Geometry check sheet. Reference: the model listing, model coordinates, mm. A direction names the side the tool comes from. Give positions to 0.01 mm unless a question says otherwise; leave off trailing zeros. Loops run counter-clockwise (first coordinate to the right, second up) from the corner with the lowest first, then second, coordinate; pieces in that order, holes last. Notation, with made-up numbers: (82, -38.75) -> (93, -38.75) arc R5 cw to (93, -29.75) -> close; hole circle Ø5 at (-31.75, -32). An arc over 180 degrees is marked (long way). Write each question's results on one line, items separated by ' | '. Start each with the question number.
1) Depth check by flat-ended pin: pin 1 (9 mm diameter, centred on x = 23, z = -14, fed in from -Y); pin 2 (1 mm diameter, centred on x = 18.5, y = -13.5, fed in from -Z); pin 3 (8 mm diameter, centred on x = 5.5, z = -12, fed in from -Y). Enter the tip coordinate at first touch or a pass-through.
2) Draft check along Z on faces 3 (the face through (18.36, -16.41, -9.74)), 4 (the face through (20, 0, -14)), 5 (the face through (18.95, -21.32, -17.1)). Enter one of: pulls with the +Z half, pulls with the -Z half, needs draft (parallel to the pull), parting line crosses it, or undercut.
3) Sectioned sample at B-B on y = -8.25. Record the cut outline in (x, z).
4) Sectioned sample at C-C on z = -14. Record the cut outline in (x, y).
5) Scan lines: line 1 (Y direction, x = 3, z = -13.5); line 2 (Y direction, x = 11.5, z = -16.5); line 3 (Z direction, x = 23, y = -20). Record each from-to range of solid material in increasing order. Write a range as from..to.
6) Sectioned sample at D-D on x = 23. Record the cut outline in (y, z).
7) Set-up check for faces 1 (the face through (0, -5, -14)), 2 (the face through (7, -7.8, -14)): record each of +Z, -Z, +X, -X, +Y, -Y from which the full face is reachable in a straight line by a thin tool's end or side.
8) Sectioned sample at A-A on x = 7. Record the cut outline in (y, z).
```python
from build123d import *

# Parameters (mm, degrees)
F0_W     = 40.5
F0_H     = 28
F1_DEPTH = 9.8
F2_R     = 6.3
F2_R_2   = 5.1
F3_DEPTH = 13.4
F4_DEPTH = 9.7
F5_R     = 5
F6_DEPTH = 2


# Not quite as in the source:
# - a feature of the source that left no trace in its solid (it failed there, or was rolled back) is left out


with BuildPart() as f1:
    # F0 (on Front) → F1 (new body)
    with BuildSketch(Plane.XZ):
        with Locations((20.25, -14)):
            Rectangle(F0_W, F0_H)
    extrude(amount=F1_DEPTH)

    # F2 (on face) → F3 (join)
    with BuildSketch(Plane.XZ.offset(9.8)):
        with Locations((23, -14)):
            Circle(F2_R)
        with Locations((23, -14)):
            Circle(F2_R_2, mode=Mode.SUBTRACT)
    extrude(amount=F3_DEPTH)

    # F4 (add): a face of the model
    f4_faces = [f1.faces().sort_by_distance(p)[0] for p in [
        (23, -9.8, -14),
    ]]
    extrude(f4_faces, amount=F4_DEPTH)

    # F5 (on face) → F6 (cut)
    with BuildSketch(Plane.XZ.offset(9.8)):
        with Locations((7, -14)):
            Circle(F5_R)
    extrude(amount=-F6_DEPTH, mode=Mode.SUBTRACT)


solid = f1.part
```
Result:
1) pin 1: y = -19.5 | pin 2: z = -18.87 | pin 3: y = -9.8
2) face 3: parting line crosses it | face 4: needs draft | face 5: undercut
3) outline: (0, -28) -> (40.5, -28) -> (40.5, 0) -> (0, 0) -> close; hole circle Ø10 at (7, -14)
4) outline: (0, -9.8) -> (2, -9.8) -> (2, -7.8) -> (12, -7.8) -> (12, -9.8) -> (16.7, -9.8) -> (16.7, -23.2) -> (17.9, -23.2) -> (17.9, -19.5) -> (28.1, -19.5) -> (28.1, -23.2) -> (29.3, -23.2) -> (29.3, -9.8) -> (40.5, -9.8) -> (40.5, 0) -> (0, 0) -> close
5) line 1: -7.8..0 | line 2: -9.8..0 | line 3: -20.3..-19.1, -8.9..-7.7
6) outline: (-23.2, -20.3) -> (-9.8, -20.3) -> (-9.8, -28) -> (0, -28) -> (0, 0) -> (-9.8, 0) -> (-9.8, -7.7) -> (-23.2, -7.7) -> (-23.2, -8.9) -> (-19.5, -8.9) -> (-19.5, -19.1) -> (-23.2, -19.1) -> close
7) face 1: +Z, -Z, -X, +Y, -Y | face 2: -Y
8) outline: (-9.8, -28) -> (0, -28) -> (0, 0) -> (-9.8, 0) -> (-9.8, -9) -> (-7.8, -9) -> (-7.8, -19) -> (-9.8, -19) -> close
